For this review, take the finished solid that the model builds, in its own axes (mm). Give positions to 0.01 mm unless a question says otherwise; leave off trailing zeros. Loops run counter-clockwise (first coordinate to the right, second up) from the corner with the lowest first, then second, coordinate; pieces in that order, holes last.
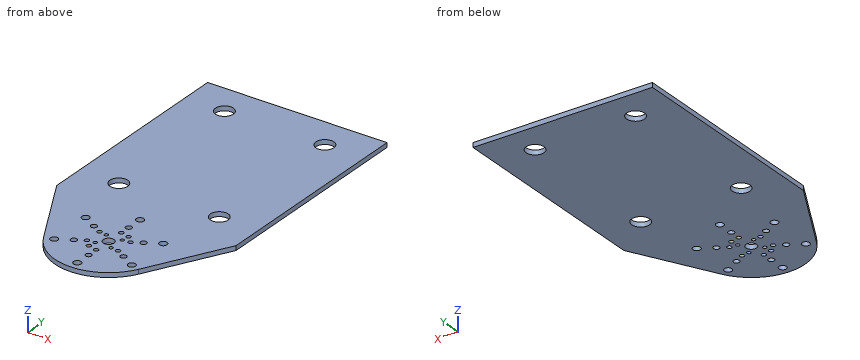
```python
from build123d import *

# Parameters (mm, degrees)
BOSS_EXTRUDE1_DEPTH        = 6.35
SIA20_80MM_X_M8_X_6_D      = 8.4
IRB2400_50MM_X_M6_X_6_D    = 6.4
UR5_50MM_X_M6_X_4_D        = 6.4
R2000_125MM_X_M10_X_6_D    = 10.5
M5_CLEARANCE_HOLE1_D       = 5.3
F_25_0_25_DIAMETER_HOLE2_D = 25
F_15_0_15_DIAMETER_HOLE1_D = 15


with BuildPart() as part:
    # Sketch1 → Boss-Extrude1 (new body)
    with BuildSketch(Plane.XY):
        with BuildLine():
            Line((-125, 375), (125, 375))
            Line((125, 375), (125, 75))
            Line((125, 75), (66.176470588, -35.294117647))
            ThreePointArc((66.176470588, -35.294117647), (0, -75), (-66.176470588, -35.294117647))
            Line((-66.176470588, -35.294117647), (-125, 75))
            Line((-125, 75), (-125, 375))
        make_face()
    extrude(amount=BOSS_EXTRUDE1_DEPTH)

    # SIA20 (80mm x M8 x 6) (through all)
    with Locations(Plane.XY.offset(6.35)):
        with Locations((-34.641016151, 20), (-34.641016151, -20), (0, -40), (34.641016151, -20), (34.641016151, 20), (0, 40)):
            Hole(SIA20_80MM_X_M8_X_6_D / 2)

    # IRB2400 (50mm x M6 x 6) (through all)
    with Locations(Plane.XY.offset(6.35)):
        with Locations((0, 25), (21.650635095, -12.5), (21.650635095, 12.5), (-21.650635095, 12.5), (-21.650635095, -12.5), (0, -25)):
            Hole(IRB2400_50MM_X_M6_X_6_D / 2)

    # UR5 (50mm x M6 x 4) (through all)
    with Locations(Plane.XY.offset(6.35)):
        with Locations((12.5, 21.650635095), (-21.650635095, 12.5), (-12.5, -21.650635095), (21.650635095, -12.5)):
            Hole(UR5_50MM_X_M6_X_4_D / 2)

    # R2000 (125mm x M10 x 6) (through all)
    with Locations(Plane.XY.offset(6.35)):
        with Locations((-54.126587737, 31.25), (0, 62.5), (54.126587737, 31.25), (54.126587737, -31.25), (0, -62.5), (-54.126587737, -31.25)):
            Hole(R2000_125MM_X_M10_X_6_D / 2)

    # M5 Clearance Hole1 (through all)
    with Locations(Plane.XY.offset(6.35)):
        with Locations((-11.136931804, 11.136931804), (11.136931804, 11.136931804), (11.136931804, -11.136931804), (-11.136931804, -11.136931804)):
            Hole(M5_CLEARANCE_HOLE1_D / 2)

    # Ø25.0 (25) Diameter Hole2 (through all)
    with Locations(Plane.XY.offset(6.35)):
        with Locations((-70, 330), (-70, 120), (70, 120), (70, 330)):
            Hole(F_25_0_25_DIAMETER_HOLE2_D / 2)

    # Ø15.0 (15) Diameter Hole1 (through all)
    with Locations(Plane.XY.offset(6.35)):
        with Locations((0, 0)):
            Hole(F_15_0_15_DIAMETER_HOLE1_D / 2)


solid = part.part
```
Item 1: Take a section at B-B on y = 0. Give the boundary of the cut face in (x, z).
Answer:
outline: (-85, 0) - (-7.5, 0) - (-7.5, 6.35) - (-85, 6.35) - close; (7.5, 0) - (85, 0) - (85, 6.35) - (7.5, 6.35) - close
Item 2: Take a section at A-A on y = 120. Give the boundary of the cut face in (x, z).
Answer:
outline: (-125, 0) - (-82.5, 0) - (-82.5, 6.35) - (-125, 6.35) - close; (-57.5, 0) - (57.5, 0) - (57.5, 6.35) - (-57.5, 6.35) - close; (82.5, 0) - (125, 0) - (125, 6.35) - (82.5, 6.35) - close
Item 3: Take a section at C-C on x = 78. Give the boundary of the cut face in (y, z) (3 decimals), and give its area (3 significant figures).
Answer:
outline: (-13.125, 0) - (110.395, 0) - (110.395, 6.35) - (-13.125, 6.35) - close; (129.605, 0) - (320.395, 0) - (320.395, 6.35) - (129.605, 6.35) - close; (339.605, 0) - (375, 0) - (375, 6.35) - (339.605, 6.35) - close
area: 2,220 mm2
Item 4: Clearance check with flat-ended pins moving along their axes: pin 1 Ø13.5 at (x, y) = (34.64, 20) entering from +Z; pin 2 Ø1 at (y, z) = (31, 1) entering from -X; pin 3 Ø3 at (x, z) = (73, 1) entering from -Y. State where each tip first meets the part, or that it passes through.
Answer:
pin 1: stops at z = 6.35
pin 2: stops at x = -101.8
pin 3: stops at y = -25.31
Item 5: For L1, parallel to Y at x = 61, z = 5.5; L2, parallel to Y at x = -73, z = 3.25; L3, parallel to X at y = 339.5, z = 1.25, list the stretches that pass through material, from the lowest coordinate up.
Answer:
L1: y = -43.63 to 111.33, 128.67 to 321.33, 338.67 to 375
L2: y = -22.5 to 107.87, 132.13 to 317.87, 342.13 to 375
L3: x = -125 to -78.12, -61.88 to 61.88, 78.12 to 125
Item 6: Take a section at D-D on y = 62.5. Give the boundary of the cut face in (x, z), and give its area (3 significant figures).
Answer:
outline: (-118.33, 0) - (-5.25, 0) - (-5.25, 6.35) - (-118.33, 6.35) - close; (5.25, 0) - (118.33, 0) - (118.33, 6.35) - (5.25, 6.35) - close
area: 1,440 mm2
